Check sheet for the modelled part. Datum: model origin and axes. Units: mm. Face numbers are marked on the shaded views. A direction names the side the tool comes from. Coordinates: 2 decimals unless noted, no trailing zeros. Loops run counter-clockwise (first coordinate to the right, second up) from the corner with the lowest first, then second, coordinate; pieces in that order, holes last.
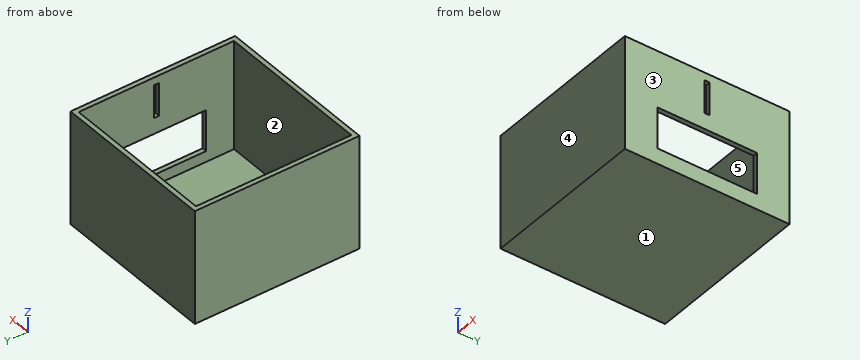
Autodesk Fusion 360 part; units mm, degrees
sketch "Sketch1" plane through (0, 0, 0) normal (0, 0, 1) x (1, 0, 0)
  line L0 (-80, 80) -> (80, 80)
  line L1 (80, 80) -> (80, -80)
  line L2 (80, -80) -> (-80, -80)
  line L3 (-80, -80) -> (-80, 80)
  line L4 (-80, 80) -> (80, -80) construction
  line L5 (80, 80) -> (-80, -80) construction
  dimension "d1" = 160
  dimension "d3" = 160
extrude "Extrude1" add sketch "Sketch1" along normal blind 110
sketch "Sketch3" plane through (0, 0, 110) normal (0, 0, 1) x (-1, 0, 0)
  line L0 (80, 80) -> (-80, 80)
  line L1 (-80, 80) -> (-80, -80)
  line L2 (-80, -80) -> (80, -80)
  line L3 (80, -80) -> (80, 80)
  line L4 (75.5, -75.5) -> (-75.5, -75.5)
  line L5 (-75.5, -75.5) -> (-75.5, 75.5)
  line L6 (-75.5, 75.5) -> (75.5, 75.5)
  line L7 (75.5, 75.5) -> (75.5, -75.5)
  line L8 (75.5, -75.5) -> (-75.5, 75.5) construction
  line L9 (-75.5, -75.5) -> (75.5, 75.5) construction
  dimension "d7" = 151
  dimension "d8" = 151
extrude "Extrude2" cut sketch "Sketch3" against normal blind 105.5 contours L4 L5 L6 L7
sketch "Sketch4" plane through (80, 0, 0) normal (1, 0, 0) x (0, 1, 0)
  line L0 (-80, 0) -> (80, 0)
  line L1 (80, 0) -> (80, 110)
  line L2 (80, 110) -> (-80, 110)
  line L3 (-80, 110) -> (-80, 0)
  line L4 (2.5, 70.5) -> (-2.5, 70.5)
  line L5 (-2.5, 70.5) -> (-2.5, 102.5)
  line L6 (-2.5, 102.5) -> (2.5, 102.5)
  line L7 (2.5, 102.5) -> (2.5, 70.5)
  line L8 (2.5, 70.5) -> (-2.5, 102.5) construction
  line L9 (-2.5, 70.5) -> (2.5, 102.5) construction
  point P0 (0, 86.5)
  dimension "d11" = 7.5
  dimension "d12" = 32
  dimension "d13" = 5
  dimension "d14" = 77.5
extrude "Extrude3" cut sketch "Sketch4" against normal blind 5 contours L4 L5 L6 L7
sketch "Sketch5" plane through (80, 0, 0) normal (1, 0, 0) x (0, 1, 0)
  line L0 (-2.5, 70.5) -> (-2.5, 102.5)
  line L1 (-2.5, 102.5) -> (2.5, 102.5)
  line L2 (2.5, 102.5) -> (2.5, 70.5)
  line L3 (2.5, 70.5) -> (-2.5, 70.5)
  line L4 (-80, 0) -> (80, 0)
  line L5 (80, 0) -> (80, 110)
  line L6 (80, 110) -> (-80, 110)
  line L7 (-80, 110) -> (-80, 0)
  line L8 (48.5, 55) -> (-48.5, 55)
  line L9 (-48.5, 55) -> (-48.5, 15)
  line L10 (-48.5, 15) -> (48.5, 15)
  line L11 (48.5, 15) -> (48.5, 55)
  line L12 (48.5, 55) -> (-48.5, 15) construction
  line L13 (-48.5, 55) -> (48.5, 15) construction
  point P0 (0, 35)
  dimension "d17" = 97
  dimension "d18" = 31.5
  dimension "d19" = 40
  dimension "d20" = 15
extrude "Extrude4" cut sketch "Sketch5" against normal blind 5 contours L8 L9 L10 L11
equation "d1 = Cube_size"
equation "d3 = Cube_size"
equation "Cube_size = 160 mm"
equation "d5 = Cube_size / 16 * 11"
equation "d7 = Cube_size - Cube_size * 0.05625"
equation "d8 = Cube_size - Cube_size * 0.05625"
equation "d9 = 0.6875 * Cube_size * 0.0409090909090909 - 0.6875 * Cube_size"
equation "d11 = 0.6875 * Cube_size * 0.0681818181818182"
equation "d12 = 0.6875 * Cube_size * 0.2909090909090909"
equation "d13 = 0.0454545454545455 * 0.6875 * Cube_size"
equation "d14 = ( Cube_size - 0.0454545454545455 * 0.6875 * Cube_size ) / 2"
equation "d15 = -Cube_size * 0.03125"
equation "d17 = Cube_size * 0.60625"
equation "d18 = Cube_size * 0.196875"
equation "d19 = 0.25 * Cube_size"
equation "d20 = Cube_size * 0.09375"
equation "d21 = -Cube_size * 0.03125"
1) Section check D-D on z = 46. Enter the section's corners in (x, y), plus the area to 3 significant figures.
Answer sheet:
outline: (-80, -80) - (80, -80) - (80, -48.5) - (75.5, -48.5) - (75.5, -75.5) - (-75.5, -75.5) - (-75.5, 75.5) - (75.5, 75.5) - (75.5, 48.5) - (80, 48.5) - (80, 80) - (-80, 80) - close
area: 2,360 mm2
2) Set-up check for the marked faces 1 and 2: record each of +Z, -Z, +X, -X, +Y, -Y from which the full face is reachable in a straight line by a thin tool's end or side.
Answer sheet:
face 1: -Z, +X, -X, +Y, -Y
face 2: +Z
3) Depth check by flat-ended pin: pin 1 (6 mm diameter, centred on x = 15, y = -0.5, fed in from +Z). Enter the tip coordinate at first touch or a pass-through.
Answer sheet:
pin 1: stops at z = 4.5
4) Section check C-C on z = 9. Enter the section's corners in (x, y).
Answer sheet:
outline: (-80, -80) - (80, -80) - (80, 80) - (-80, 80) - close; hole (-75.5, -75.5) - (75.5, -75.5) - (75.5, 75.5) - (-75.5, 75.5) - close
5) Section check B-B on x = 31.5. Enter the section's corners in (y, z).
Answer sheet:
outline: (-80, 0) - (80, 0) - (80, 110) - (75.5, 110) - (75.5, 4.5) - (-75.5, 4.5) - (-75.5, 110) - (-80, 110) - close
6) Scan lines: line 1 (Y direction, x = 44.5, z = 56.5); line 2 (X direction, y = 8, z = 27). Record each from-to range of solid material in increasing order.
Answer sheet:
line 1: y = -80 to -75.5, 75.5 to 80
line 2: x = -80 to -75.5
7) Mould release check, pull along X, two halves, no side actions. Record for the marked faces 3, 4 and 5: +X half, -X half, draft (parallel to the pull), parting line (faces both ways), or undercut.
Answer sheet:
face 3: +X half
face 4: draft
face 5: undercut
8) Section check A-A on y = -13. Enter the section's corners in (x, z), plus the area to 3 significant figures.
Answer sheet:
outline: (-80, 0) - (80, 0) - (80, 15) - (75.5, 15) - (75.5, 4.5) - (-75.5, 4.5) - (-75.5, 110) - (-80, 110) - close; (75.5, 55) - (80, 55) - (80, 110) - (75.5, 110) - close
area: 1,490 mm2
